Study the drawing (mm; zero at the part's minimum x, y, z) and answer. A direction names the side the tool comes from. Give positions to 0.01 mm unless a question says otherwise; leave off trailing zeros. Order: outer loops, then holes, each group sorted by start corner. A loop starts at its lowest first (then second) coordinate and runs counter-clockwise, first axis right, second up. Notation, with made-up numbers: (44.5, -12) - (93.5, -12) arc R24 cw to (93.5, 10) - close; hole circle Ø6 at (79.25, 14). An arc over 180 degrees is marked (long way). Put each result on its own line as item: value.
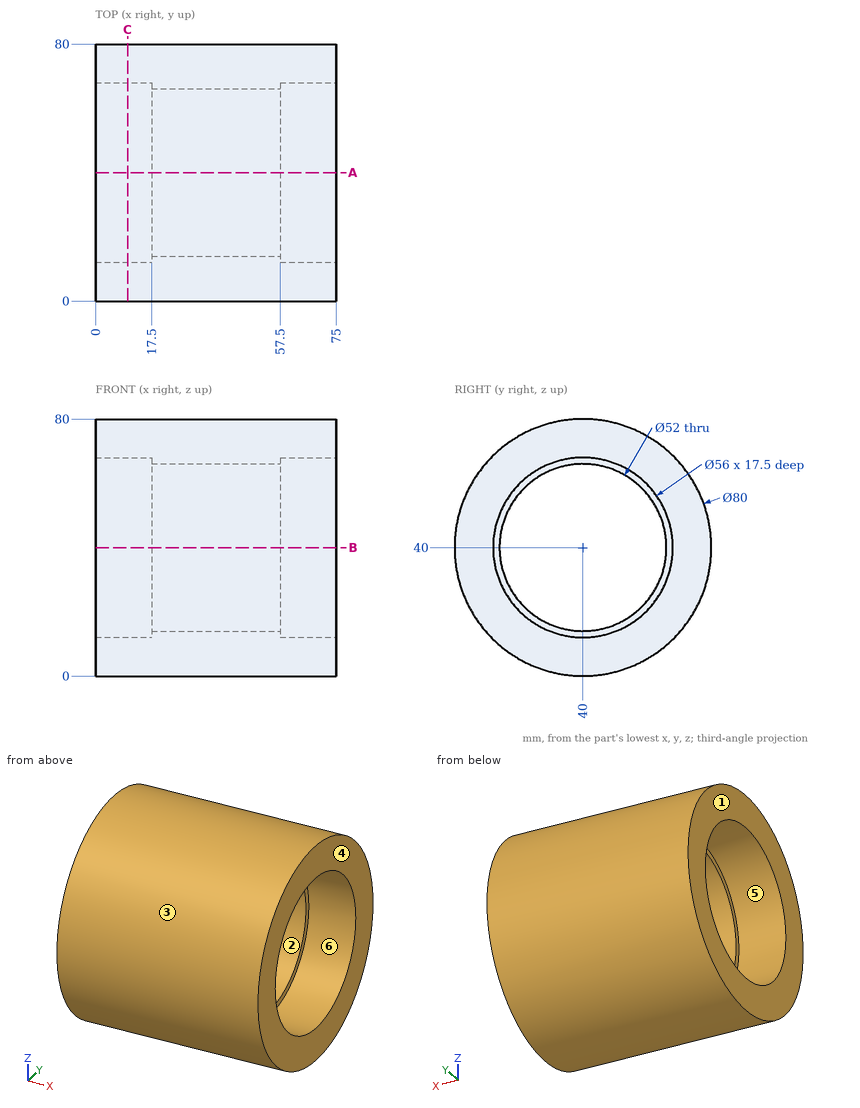
(1) Section A-A, the plane y = 40 is taken. Write down the section's boundary in (x, z), then the cut area to 3 significant figures.
Geometry check:
outline: (0, 0) - (75, 0) - (75, 12) - (57.5, 12) - (57.5, 14) - (17.5, 14) - (17.5, 12) - (0, 12) - close; (0, 68) - (17.5, 68) - (17.5, 66) - (57.5, 66) - (57.5, 68) - (75, 68) - (75, 80) - (0, 80) - close
area: 1,960 mm²
(2) Determine the mould class of the marked faces 1, 2 and 3 for opening direction Z: pulls with the +Z half, pulls with the -Z half, needs draft (parallel to the pull), parting line crosses it, or undercut.
Geometry check:
face 1: needs draft
face 2: undercut
face 3: parting line crosses it
(3) Straight lines are drawn through the part: line 1 (Z direction, x = 68, y = 40); line 2 (Z direction, x = 12.5, y = 47.5); line 3 (Y direction, x = 20.5, z = 41). For each, find the intervals that lie inside material, in ascending order.
Geometry check:
line 1: z = 0 to 12, 68 to 80
line 2: z = 0.71 to 13.02, 66.98 to 79.29
line 3: y = 0.01 to 14.02, 65.98 to 79.99
(4) Given pin 1 (2 mm diameter, centred on x = 63, y = 42.5, fed in from -Z); pin 2 (1 mm diameter, centred on x = 49, y = 49.5, fed in from -Z); pin 3 (17 mm diameter, centred on y = 51, z = 34.5, fed in from -X); pin 4 (1 mm diameter, centred on x = 59.5, z = 27.5, fed in from +Y), each flat-ended and moving along its own axis, determine where each tip first touches the part or whether it passes through.
Geometry check:
pin 1: stops at z = 0.03
pin 2: stops at z = 1.03
pin 3: passes through
pin 4: stops at y = 78.16
(5) Section C-C, the plane x = 10 is taken. Write down the section's boundary in (y, z), then the cut area to 3 significant figures.
Geometry check:
outline: circle Ø80 at (40, 40); hole circle Ø56 at (40, 40)
area: 2,560 mm²
(6) A tool of negligible diameter and unlimited length cuts with its end or side. For the marked faces 4, 5 and 6, from which of +Z, -Z, +X, -X, +Y, -Y can it reach the whole face along a straight path? Write none if from no direction.
Geometry check:
face 4: +Z, -Z, +X, +Y, -Y
face 5: -X
face 6: +X
